Build history of the part. All positions in model axes, mm. Face numbers are marked on the shaded views. A direction names the side the tool comes from. Give positions to 0.01 mm unless a question says otherwise; leave off trailing zeros. Write each loop counter-clockwise with the first axis right and the second up, starting at its lowest first coordinate (ties: lowest second). Pieces come first, ordered by that corner, then holes.
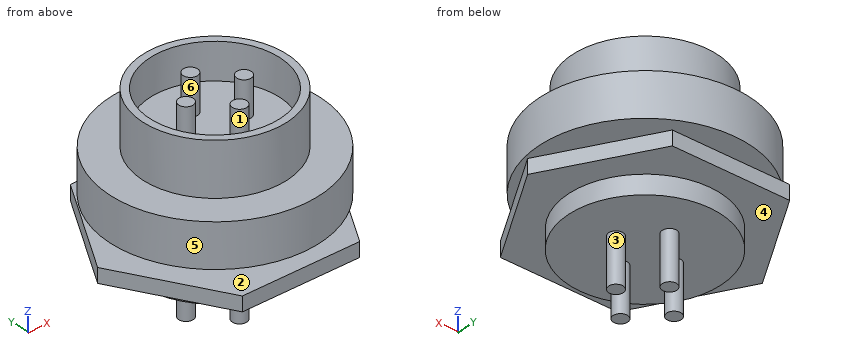
from build123d import *

# Parameters (mm, degrees)
DODANIE_WYCI_GNI_CIE1_DEPTH       = 2.4
SZKIC2_R                          = 14.5
DODANIE_WYCI_GNI_CIE2_DEPTH       = 6
SZKIC3_R                          = 10
DODANIE_WYCI_GNI_CIE3_DEPTH       = 7.3
DODANIE_WYCI_GNI_CIE4_START       = -5
DODANIE_WYCI_GNI_CIE4_OUTLINE_R   = 9
DODANIE_WYCI_GNI_CIE4_OUTLINE_R_2 = 1
DODANIE_WYCI_GNI_CIE4_DEPTH       = 5
DODANIE_WYCI_GNI_CIE5_DEPTH       = 2
DODANIE_WYCI_GNI_CIE6_START       = 7
SZKIC6_R                          = 10.5
DODANIE_WYCI_GNI_CIE6_DEPTH       = 2.6
DODANIE_WYCI_GNI_CIE7_START       = 6.7
SZKIC7_R                          = 1
DODANIE_WYCI_GNI_CIE7_DEPTH       = 6.7


# Read off the part's stored shape, not the designer's step: Dodanie-wyciągnięcie4
with BuildPart() as part:
    # Szkic1 → Dodanie-wyciągnięcie1 (new body)
    with BuildSketch(Plane.XY):
        with BuildLine():
            Line((-4.019950248, 9.7), (4.019950248, 9.7))
            ThreePointArc((4.019950248, 9.7), (0, -10.5), (-4.019950248, 9.7))
        make_face()
    extrude(amount=DODANIE_WYCI_GNI_CIE1_DEPTH)

    # Szkic2 → Dodanie-wyciągnięcie2 (add)
    with BuildSketch(Plane.XY.offset(2.4)):
        Circle(SZKIC2_R)
    extrude(amount=DODANIE_WYCI_GNI_CIE2_DEPTH)

    # Szkic3 → Dodanie-wyciągnięcie3 (add)
    with BuildSketch(Plane.XY.offset(8.4)):
        with Locations(Location((0, 0, 0), (0, 0, 180))):
            Circle(SZKIC3_R)
    extrude(amount=DODANIE_WYCI_GNI_CIE3_DEPTH)

    # Dodanie-wyciągnięcie4 outline → Dodanie-wyciągnięcie4 (cut)
    with BuildSketch(Plane.XY.offset(15.7).offset(DODANIE_WYCI_GNI_CIE4_START)):
        Circle(DODANIE_WYCI_GNI_CIE4_OUTLINE_R)
        with Locations((0, -4)):
            Circle(DODANIE_WYCI_GNI_CIE4_OUTLINE_R_2, mode=Mode.SUBTRACT)
        with Locations((-4, 0)):
            Circle(DODANIE_WYCI_GNI_CIE4_OUTLINE_R_2, mode=Mode.SUBTRACT)
        with Locations((4, 0)):
            Circle(DODANIE_WYCI_GNI_CIE4_OUTLINE_R_2, mode=Mode.SUBTRACT)
        with Locations((0, 4)):
            Circle(DODANIE_WYCI_GNI_CIE4_OUTLINE_R_2, mode=Mode.SUBTRACT)
    extrude(amount=DODANIE_WYCI_GNI_CIE4_DEPTH, mode=Mode.SUBTRACT)

    # Szkic5 → Dodanie-wyciągnięcie5 (add)
    with BuildSketch(Plane(origin=(0, 0, 0), x_dir=(-1, 0, 0), z_dir=(0, 0, -1))):
        Polygon((8.082903769, 14), (-8.082903769, 14), (-16.165807537, 0), (-8.082903769, -14), (8.082903769, -14), (16.165807537, 0), align=None)
    extrude(amount=DODANIE_WYCI_GNI_CIE5_DEPTH)

    # Szkic6 → Dodanie-wyciągnięcie6 (add)
    with BuildSketch(Plane(origin=(0, 0, 2.4), x_dir=(-1, 0, 0), z_dir=(0, 0, -1)).offset(DODANIE_WYCI_GNI_CIE6_START)):
        Circle(SZKIC6_R)
    extrude(amount=-DODANIE_WYCI_GNI_CIE6_DEPTH)

    # Szkic7 → Dodanie-wyciągnięcie7 (add)
    with BuildSketch(Plane(origin=(0, 0, -4.6), x_dir=(-1, 0, 0), z_dir=(0, 0, -1)).offset(DODANIE_WYCI_GNI_CIE7_START)):
        with Locations(Location((0, -4, 0), (0, 0, 180))):
            Circle(SZKIC7_R)
        with Locations(Location((4, 0, 0), (0, 0, 180))):
            Circle(SZKIC7_R)
        with Locations(Location((0, 4, 0), (0, 0, 180))):
            Circle(SZKIC7_R)
        with Locations(Location((-4, 0, 0), (0, 0, 180))):
            Circle(SZKIC7_R)
    extrude(amount=-DODANIE_WYCI_GNI_CIE7_DEPTH)


solid = part.part
1. Drill centre lines: line 1 along Y through (x, z) = (0, 13.5); line 2 along Z through (x, y) = (-11.5, 0.5); line 3 along Z through (x, y) = (0.5, 0.5). Where is each one in solid material? Low to high.
2. Saw through at C-C on z = 1. Give the cut face in (x, y).
3. Saw through at A-A on y = 11.75. Give the cut face in (x, z).
4. Drop flat-ended pins along their axis: pin 1 (8 mm diameter, centred on y = 10, z = -7, fed in from +X); pin 2 (1.5 mm diameter, centred on x = 7.5, y = 10.5, fed in from +Z); pin 3 (2 mm diameter, centred on y = -7, z = -4, fed in from -X); pin 4 (1 mm diameter, centred on x = -12.5, z = -3, fed in from +Y). Give the stop position or say it passes through.
5. Saw through at B-B on x = 12. Give the cut face in (y, z), plus the area to 3 significant figures.
6. Mould opens along X. For the marked faces 4, 5 and 6 say: pulls with the +X half, pulls with the -X half, needs draft (parallel to the pull), parting line crosses it, or undercut.
7. 3-axis set-ups, long thin cutter, end or side, ignore diameter. For the marked faces 1, 2 and 3: which of +Z, -Z, +X, -X, +Y, -Y reach the whole face in a straight line?
Outcome:
1. line 1: y = -10 to -9, -5 to -3, 3 to 5, 9 to 10
1. line 2: z = -2 to 0, 2.4 to 8.4
1. line 3: z = -4.6 to 10.7
2. outline: (-4.02, 9.7) arc R10.5 ccw (long way) to (4.02, 9.7) - close
3. outline: (-9.38, -2) - (9.38, -2) - (9.38, 0) - (-9.38, 0) - close; (-8.5, 2.4) - (8.5, 2.4) - (8.5, 8.4) - (-8.5, 8.4) - close
4. pin 1: stops at x = 8
4. pin 2: stops at z = 8.4
4. pin 3: stops at x = -8.62
4. pin 4: passes through
5. outline: (-8.14, 2.4) - (8.14, 2.4) - (8.14, 8.4) - (-8.14, 8.4) - close; (-7.22, -2) - (7.22, -2) - (7.22, 0) - (-7.22, 0) - close
5. area: 127 mm2
6. face 4: needs draft
6. face 5: parting line crosses it
6. face 6: undercut
7. face 1: +Z
7. face 2: none
7. face 3: -Z
